```python
from build123d import *

# Parameters (mm, degrees)
CROQUIS1_R              = 1.5
SALIENTE_EXTRUIR1_DEPTH = 10
CROQUIS2_R              = 2.5
SALIENTE_EXTRUIR2_DEPTH = 45


with BuildPart() as part:
    # Croquis1 → Saliente-Extruir1 (new body)
    with BuildSketch(Plane.XY):
        with BuildLine():
            Line((-5, 0), (-5, -5))
            Line((-5, -5), (5, -5))
            Line((5, -5), (5, 0))
            ThreePointArc((5, 0), (0, 5), (-5, 0))
        make_face()
        Circle(CROQUIS1_R, mode=Mode.SUBTRACT)
    extrude(amount=SALIENTE_EXTRUIR1_DEPTH)

    # Croquis2 → Saliente-Extruir2 (add)
    with BuildSketch(Plane.XZ.offset(5)):
        with Locations(Location((0, 5, 0), (0, 0, 90))):
            Circle(CROQUIS2_R)
    extrude(amount=SALIENTE_EXTRUIR2_DEPTH)


solid = part.part
```
Verification items for the finished model (mm, model axes). A direction names the side the tool comes from. Coordinates: 2 decimals unless noted, no trailing zeros. Loops run counter-clockwise (first coordinate to the right, second up) from the corner with the lowest first, then second, coordinate; pieces in that order, holes last. Notation, with made-up numbers: (-26, 33) - (-13, 33) arc R10 ccw to (-13, 44) - close; hole circle Ø6 at (5, 63.5). An arc over 180 degrees is marked (long way). Answer as a JSON object with one key per item and string values.
(1) Scan lines: line 1 along Y through (x, z) = (0, 8); line 2 along X through (y, z) = (-11.5, 5); line 3 along Y through (x, z) = (0, 3.5). Record each from-to range of solid material in increasing order.
Response:
{"line 1": "y = -5 to -1.5, 1.5 to 5", "line 2": "x = -2.5 to 2.5", "line 3": "y = -50 to -1.5, 1.5 to 5"}
(2) Cross-section at A-A, the plane z = 6.5. Record the boundary of the cut face in (x, y), then the cut area to 3 significant figures.
Response:
{"outline": "(-5, -5) - (-2, -5) - (-2, -50) - (2, -50) - (2, -5) - (5, -5) - (5, 0) arc R5 ccw to (-5, 0) - close; hole circle Ø3 at (0, 0)", "area": "262 mm²"}
(3) Mould release check, pull along Y, two halves, no side actions. Record for faces 1 (the flat face through (0, -50, 5)), 2 (the cylindrical face through (-1.5, 0.07, 4.93)), 3 (the flat face through (-5, -2, 5)): pulls with the +Y half, pulls with the -Y half, needs draft (parallel to the pull), parting line crosses it, or undercut.
Response:
{"face 1": "pulls with the -Y half", "face 2": "undercut", "face 3": "needs draft"}
(4) Go/stop test with flat-tipped pins: pin 1 Ø4 at (x, y) = (0.5, -19.5) entering from -Z; pin 2 Ø1 at (x, z) = (3.5, 5) entering from -Y; pin 3 Ø1 at (y, z) = (-13, 5.5) entering from +X. Record where each tip stops, or that it passes through.
Response:
{"pin 1": "stops at z = 2.5", "pin 2": "stops at y = -5", "pin 3": "stops at x = 2.5"}
(5) Cross-section at D-D, the plane y = -34. Record the boundary of the cut face in (x, z), then the cut area to 3 significant figures.
Response:
{"outline": "circle Ø5 at (0, 5)", "area": "19.6 mm²"}
(6) Access from +Z, -Z, +X, -X, +Y, -Y to the whole of each face (thin tool, end or side, straight path). Record for faces 4 (the flat face through (0, -2, 0)), 5 (the flat face through (-2, -5, 3)).
Response:
{"face 4": "-Z, +X, -X, +Y, -Y", "face 5": "-Y"}
(7) Cross-section at B-B, the plane x = 0. Record the boundary of the cut face in (y, z), then the cut area to 3 significant figures.
Response:
{"outline": "(-50, 2.5) - (-5, 2.5) - (-5, 0) - (-1.5, 0) - (-1.5, 10) - (-5, 10) - (-5, 7.5) - (-50, 7.5) - close; (1.5, 0) - (5, 0) - (5, 10) - (1.5, 10) - close", "area": "295 mm²"}
(8) Cross-section at C-C, the plane x = 4. Record the boundary of the cut face in (y, z), then the cut area to 3 significant figures.
Response:
{"outline": "(-5, 0) - (3, 0) - (3, 10) - (-5, 10) - close", "area": "80.0 mm²"}
